```python
from build123d import *

# Parameters (mm, degrees)
SKETCH_1_R          = 2.1
SKETCH_1_W          = 5
SKETCH_1_H          = 7
SKETCH_1_W_2        = 7
SKETCH_1_H_2        = 5
SKETCH_1_W_3        = 19.5
SKETCH_1_H_3        = 6.75
EXTRUDE_2_DEPTH     = 6
SKETCH_2_R          = 1.6
CUT_EXTRUDE_1_DEPTH = 5
SKETCH_3_R          = 1.6
CUT_EXTRUDE_2_DEPTH = 5
SKETCH_4_R          = 1.6
CUT_EXTRUDE_3_DEPTH = 5
SKETCH_5_R          = 1.6
CUT_EXTRUDE_4_DEPTH = 5
EXTRUDE_3_DEPTH     = 6
SKETCH_7_R          = 1.6
CUT_EXTRUDE_5_DEPTH = 10
SKETCH_8_W          = 19.5
SKETCH_8_H          = 40.4
SKETCH_8_H_2        = 1
CUT_EXTRUDE_6_DEPTH = 10


with BuildPart() as part:
    # 草图1 → 凸台-拉伸2 (new body)
    # profile 1 of 6: a face of its own
    with BuildSketch(Plane.XY):
        Polygon((-9.5, 39.997474683), (-39.997474683, 9.5), (-39.997474683, 2.5), (-39.997474683, -2.5), (-39.997474683, -9.5), (-9.5, -39.997474683), (-2.5, -39.997474683), (2.5, -39.997474683), (9.5, -39.997474683), (39.997474683, -9.5), (39.997474683, -2.5), (39.997474683, 2.5), (39.997474683, 9.5), (9.5, 39.997474683), (2.5, 39.997474683), (-2.5, 39.997474683), align=None)
        Polygon((-9.75, -30.1), (-9.75, 10.3), (9.75, 10.3), (9.75, -30.1), (9.75, -36.85), (-9.75, -36.85), align=None, mode=Mode.SUBTRACT)
        with Locations((-5, 14.465)):
            Circle(SKETCH_1_R, mode=Mode.SUBTRACT)
        with Locations((5, 14.465)):
            Circle(SKETCH_1_R, mode=Mode.SUBTRACT)
    # profile 2 of 6: a face of its own
    with BuildSketch(Plane.XY):
        with Locations((0, 43.497474683)):
            Rectangle(SKETCH_1_W, SKETCH_1_H)
    # profile 3 of 6: a face of its own
    with BuildSketch(Plane.XY):
        with Locations((-43.497474683, 0)):
            Rectangle(SKETCH_1_W_2, SKETCH_1_H_2)
    # profile 4 of 6: a face of its own
    with BuildSketch(Plane.XY):
        with Locations((0, -43.497474683)):
            Rectangle(SKETCH_1_W, SKETCH_1_H)
    # profile 5 of 6: a face of its own
    with BuildSketch(Plane.XY):
        with Locations((43.497474683, 0)):
            Rectangle(SKETCH_1_W_2, SKETCH_1_H_2)
    # profile 6 of 6: a face of its own
    with BuildSketch(Plane.XY):
        with Locations((0, -33.475)):
            Rectangle(SKETCH_1_W_3, SKETCH_1_H_3)
        with Locations((5, -34.165)):
            Circle(SKETCH_1_R, mode=Mode.SUBTRACT)
        with Locations((-5, -34.165)):
            Circle(SKETCH_1_R, mode=Mode.SUBTRACT)
    extrude(amount=EXTRUDE_2_DEPTH)

    # 草图2 → 切除-拉伸1 (cut)
    with BuildSketch(Plane.XZ.offset(2.5)):
        with Locations((-43.997474683, 3)):
            Circle(SKETCH_2_R)
    extrude(amount=-CUT_EXTRUDE_1_DEPTH, mode=Mode.SUBTRACT)

    # 草图3 → 切除-拉伸2 (cut)
    with BuildSketch(Plane(origin=(2.5, 0, 0), x_dir=(0, 0, -1), z_dir=(1, 0, 0))):
        with Locations(Location((-3, -43.997474683, 0), (0, 0, 90))):
            Circle(SKETCH_3_R)
    extrude(amount=-CUT_EXTRUDE_2_DEPTH, mode=Mode.SUBTRACT)

    # 草图4 → 切除-拉伸3 (cut)
    with BuildSketch(Plane(origin=(0, 2.5, 0), x_dir=(1, 0, 0), z_dir=(0, 1, 0))):
        with Locations(Location((43.997474683, -3, 0), (0, 0, 180))):
            Circle(SKETCH_4_R)
    extrude(amount=-CUT_EXTRUDE_3_DEPTH, mode=Mode.SUBTRACT)

    # 草图5 → 切除-拉伸4 (cut)
    with BuildSketch(Plane.ZY.offset(2.5)):
        with Locations(Location((3, 43.997474683, 0), (0, 0, 270))):
            Circle(SKETCH_5_R)
    extrude(amount=-CUT_EXTRUDE_4_DEPTH, mode=Mode.SUBTRACT)

    # 草图6 → 凸台-拉伸3 (add)
    with BuildSketch(Plane.XY.offset(6)):
        Polygon((-26.870057685, -31.112698372), (-22.627416998, -26.870057685), (-26.870057685, -22.627416998), (-31.112698372, -26.870057685), align=None)
    extrude(amount=-EXTRUDE_3_DEPTH)

    # 草图7 → 切除-拉伸5 (cut)
    with BuildSketch(Plane(origin=(-2.121320344, 2.121320344, 0), x_dir=(0, 0, 1), z_dir=(-0.7071067811865485, 0.7071067811865466, 0))):
        with Locations(Location((3, -38, 0), (0, 0, 270))):
            Circle(SKETCH_7_R)
    extrude(amount=-CUT_EXTRUDE_5_DEPTH, mode=Mode.SUBTRACT)

    # 草图8 → 切除-拉伸6 (cut)
    with BuildSketch(Plane(origin=(0, 0, 0), x_dir=(-1, 0, 0), z_dir=(0, 0, -1))):
        with Locations((0, -9.9)):
            Rectangle(SKETCH_8_W, SKETCH_8_H)
        with Locations((0, 10.8)):
            Rectangle(SKETCH_8_W, SKETCH_8_H_2)
        with Locations((0, -30.6)):
            Rectangle(SKETCH_8_W, SKETCH_8_H_2)
    extrude(amount=-CUT_EXTRUDE_6_DEPTH, mode=Mode.SUBTRACT)


solid = part.part
```
For this review, take the finished solid that the model builds, in its own axes (mm). A direction names the side the tool comes from. Give positions to 0.01 mm unless a question says otherwise; leave off trailing zeros. Order: outer loops, then holes, each group sorted by start corner. A loop starts at its lowest first (then second) coordinate and runs counter-clockwise, first axis right, second up.
1) Insertion check: pin 1 (3.5 mm diameter, centred on x = 5, y = -34.165, fed in from -Z); pin 2 (1.5 mm diameter, centred on x = -5, z = 5, fed in from +Y); pin 3 (2 mm diameter, centred on y = 11, z = 2, fed in from -X); pin 4 (1 mm diameter, centred on y = 5.5, z = 3.5, fed in from -X). Each pin has a flat end and moves straight along its axis. Give the tip position at first contact, or say it passes through.
2) For faces 1 (the face through (0, 11.3, 3)), 2 (the face through (42, 2.5, 3)), 3 (the face through (-16.2, -33.3, 3)), 4 (the face through (-33.5, -16, 3)), 5 (the face through (-6, -39.997, 3)), list the 3-axis set-ups (+Z, -Z, +X, -X, +Y, -Y) from which the entire face can be reached by the end or side of a thin tool; tool diameter is ignored.
3) Take a section at C-C (z = 3). State how many separate pieces and enclosed holes the cut face has, then the cut area to 3 significant figures.
4) Take a section at B-B (x = 0). Give the boundary of the cut face in (y, z), then the cut area to 3 significant figures.
5) Wall thickness on line 1 (Y direction, x = -5, z = 4.3) (3 decimals); line 2 (X direction, y = 3.5, z = 1.7); line 3 (X direction, y = -26, z = 1.65): over which ranges is each line inside the solid? List them lowest first.
6) The part is to be moulded in two halves that separate along Y. For faces 6 (the face through (0.04, -42.47, 3.48)), 7 (the face through (-6, 39.997, 3)), 8 (the face through (-11, 1, 6)), say which applies: released by +Y, released by -Y, zero draft, split by the parting line, or undercut.
7) Take a section at D-D (x = 13.5). Give the boundary of the cut face in (y, z).
8) Take a section at A-A (y = 6). Give the boundary of the cut face in (x, z), then the cut area to 3 significant figures.
Derived:
1. pin 1: passes through
1. pin 2: stops at y = 40
1. pin 3: stops at x = -39.5
1. pin 4: stops at x = -40
2. face 1: +Z, -Z
2. face 2: +Z, -Z, +X, +Y
2. face 3: +Z, -Z, -Y
2. face 4: +Z, -Z, -X
2. face 5: +Z, -Z, -X, -Y
3. separate pieces: 6
3. enclosed holes: 5
3. area: 3,750 mm2
4. outline: (-47, 0) - (-31.1, 0) - (-31.1, 6) - (-47, 6) - close; (11.3, 0) - (47, 0) - (47, 6) - (11.3, 6) - close; hole circle Ø3.2 at (-44, 3); hole circle Ø3.2 at (44, 3)
4. area: 293 mm2
5. line 1: y = -39.997 to -36.265, -32.065 to -31.1, 11.3 to 12.365, 16.565 to 39.997
5. line 2: x = -40 to -9.75, 9.75 to 40
5. line 3: x = -30.24 to -28.95, -26.53 to -9.75, 9.75 to 23.5
6. face 6: undercut
6. face 7: released by +Y
6. face 8: zero draft
7. outline: (-36, 0) - (36, 0) - (36, 6) - (-36, 6) - close
8. outline: (-40, 0) - (-9.75, 0) - (-9.75, 6) - (-40, 6) - close; (9.75, 0) - (40, 0) - (40, 6) - (9.75, 6) - close
8. area: 363 mm2
